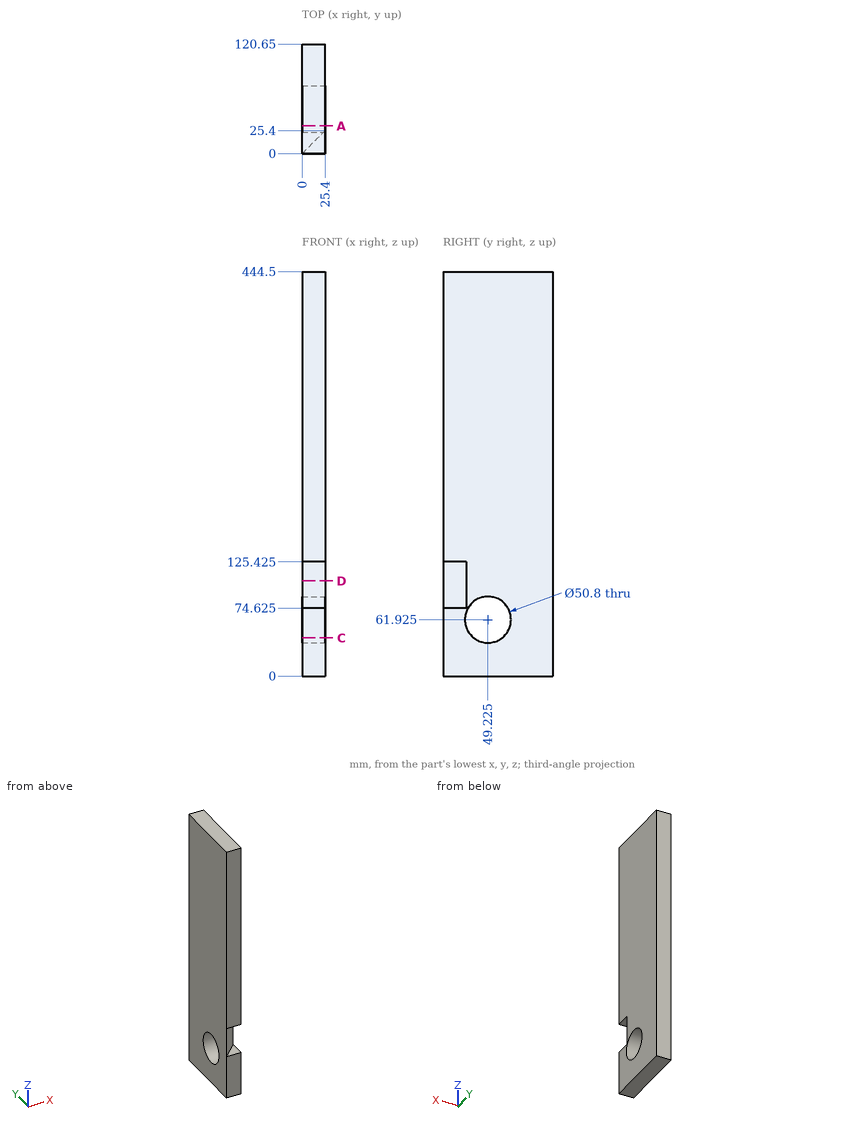
Could you check a few things on this drawing? It's one solid part, dimensions in mm from its lowest x, y, z. Round coordinates to 2 decimals unless told otherwise and drop trailing zeros. Write each loop counter-clockwise with the first axis right and the second up, starting at its lowest first coordinate (ties: lowest second). Pieces come first, ordered by that corner, then holes. Notation, with made-up numbers: (64, 43.5) -> (90, 43.5) arc R27 cw to (90, 69.5) -> close; hole circle Ø9 at (79.5, -25.5). An arc over 180 degrees is marked (long way). Use a Markdown table: item, result.
1. For pin 1 Ø8 at (y, z) = (50, 85.5) entering from +X, with a flat end and sliding along its axis, tell me the tip position at first contact or that it passes through.
Answer key:
| item | result |
|---|---|
| pin 1 | stops at x = 25.4 |
2. If we section it at A-A (y = 30.5): List the corners of the cut face in (x, z) for me.
Answer key:
| item | result |
|---|---|
| outline | (0, 0) -> (25.4, 0) -> (25.4, 44.76) -> (0, 44.76) -> close; (0, 79.09) -> (25.4, 79.09) -> (25.4, 444.5) -> (0, 444.5) -> close |
3. If we section it at D-D (z = 104.5): List the corners of the cut face in (x, y) for me.
Answer key:
| item | result |
|---|---|
| outline | (0, 0) -> (25.4, 25.4) -> (25.4, 120.65) -> (0, 120.65) -> close |
4. If we section it at C-C (z = 42): List the corners of the cut face in (x, y) for me, then the cut area to 3 significant figures.
Answer key:
| item | result |
|---|---|
| outline | (0, 0) -> (25.4, 0) -> (25.4, 33.47) -> (0, 33.47) -> close; (0, 64.98) -> (25.4, 64.98) -> (25.4, 120.65) -> (0, 120.65) -> close |
| area | 2,260 mm^2 |
5. Please list where these lines run through material, in increasing order: probe 1 along Z at (x, y) = (11, 51); probe 2 along Z at (x, y) = (22, 19) (1 decimal); probe 3 along Y at (x, z) = (15.25, 78).
Answer key:
| item | result |
|---|---|
| probe 1 | z = 0 to 36.59, 87.26 to 444.5 |
| probe 2 | z = 0 to 74.6, 125.4 to 444.5 |
| probe 3 | y = 15.25 to 29.56, 68.89 to 120.65 |
